Geometry check sheet. Reference: drawing and pictorial views, mm from the part's lowest x, y, z. Round coordinates to 2 decimals unless told otherwise and drop trailing zeros. Order: outer loops, then holes, each group sorted by start corner. A loop starts at its lowest first (then second) coordinate and runs counter-clockwise, first axis right, second up. Notation, with made-up numbers: (-30, -2.5) -> (15, -2.5) arc R22 ccw to (15, 33.5) -> close; hole circle Ø6 at (78.5, 37). An arc over 180 degrees is marked (long way). Return JSON: item names as keys, results as strings. Group by question number.
1) Section check B-B on x = 15. Enter the section's corners in (y, z).
2) Section check C-C on z = 15. Enter the section's corners in (x, y).
3) Scan lines: L1, parallel to X at y = 7.5, z = 15; L2, parallel to Z at x = 15, y = 7.25; L3, parallel to X at y = 3.75, z = 16.75 (1 decimal). Record each from-to range of solid material in increasing order.
4) Depth check by flat-ended pin: pin 1 (5 mm diameter, centred on x = 136, y = 4, fed in from -Z); pin 2 (8 mm diameter, centred on x = 131, z = 25, fed in from -Y); pin 3 (1.5 mm diameter, centred on y = 7.5, z = 21, fed in from -X); pin 4 (5 mm diameter, centred on x = 108.5, y = 5, fed in from +Z). Enter the tip coordinate at first touch or a pass-through.
5) Section check A-A on y = 3. Enter the section's corners in (x, z), plus the area to 3 significant figures.
6) Section check D-D on x = 91. Enter the section's corners in (y, z), plus the area to 3 significant figures.
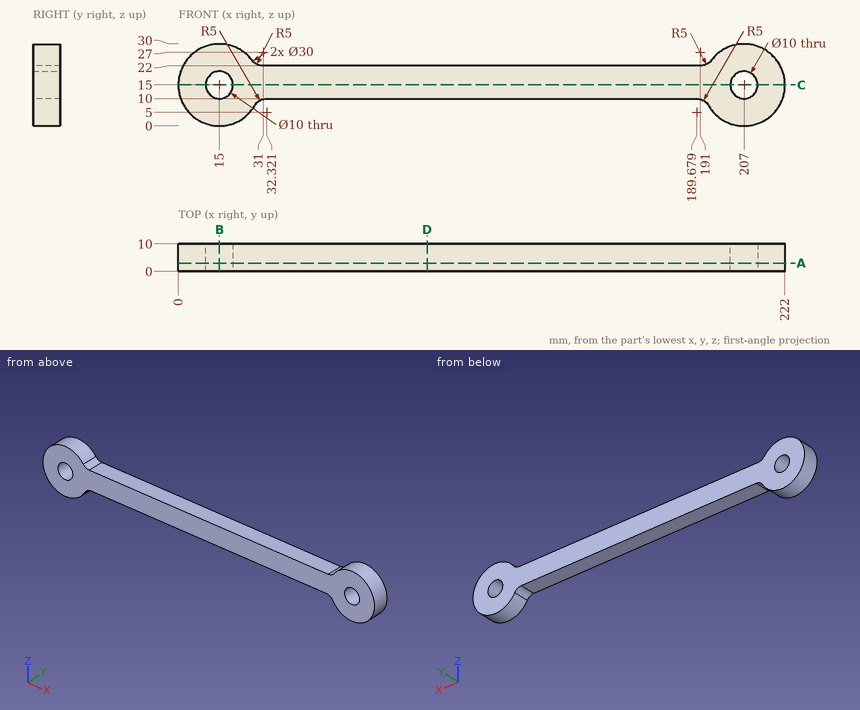
Check result:
{
 "1": {"outline": "(0, 0) -> (10, 0) -> (10, 10) -> (0, 10) -> close; (0, 20) -> (10, 20) -> (10, 30) -> (0, 30) -> close"},
 "2": {"outline": "(0, 0) -> (10, 0) -> (10, 10) -> (0, 10) -> close; (20, 0) -> (202, 0) -> (202, 10) -> (20, 10) -> close; (212, 0) -> (222, 0) -> (222, 10) -> (212, 10) -> close"},
 "3": {"L1": "0 to 10, 20 to 202, 212 to 222", "L2": "0 to 10, 20 to 30", "L3": "0.1 to 10.3, 19.7 to 202.3, 211.7 to 221.9"},
 "4": {"pin 1": "z = 10", "pin 2": "y = 0", "pin 3": "x = 0.95", "pin 4": "z = 22"},
 "5": {"outline": "(27, 24) arc R15 ccw (long way) to (27.99, 7.5) arc R5 cw to (32.32, 10) -> (189.68, 10) arc R5 cw to (194.01, 7.5) arc R15 ccw (long way) to (195, 24) arc R5 cw to (191, 22) -> (31, 22) arc R5 cw to start; hole circle Ø10 at (15, 15); hole circle Ø10 at (207, 15)", "area": "3,220 mm^2"},
 "6": {"outline": "(0, 10) -> (10, 10) -> (10, 22) -> (0, 22) -> close", "area": "120 mm^2"}
}
